Verification items for the finished model (mm, model axes). A direction names the side the tool comes from. Round coordinates to 2 decimals unless told otherwise and drop trailing zeros. Write each loop counter-clockwise with the first axis right and the second up, starting at its lowest first coordinate (ties: lowest second). Pieces come first, ordered by that corner, then holes. Notation, with made-up numbers: M -22.75,38.25 L -11.75,38.25 A18 cw -11.75,45.25 Z; hole C 9,23.5 d9. An arc over 180 degrees is marked long. Write each question's results on one line, items separated by ' | '.
from build123d import *

# Parameters (mm, degrees)
ESQUISSE1_W             = 55
ESQUISSE1_H             = 26
BOSS_EXTRU_1_DEPTH      = 25
ENL_V_MAT_EXTRU_1_REACH = 49.007
ESQUISSE2_W             = 10
ESQUISSE2_H             = 2
ENL_V_MAT_EXTRU_5_REACH = 64.857
ESQUISSE5_R             = 2.5
ESQUISSE5_W             = 26
ESQUISSE5_H             = 3.5


with BuildPart() as part:
    # Esquisse1 → Boss.-Extru.1 (new body)
    with BuildSketch(Plane(origin=(0, 0, 0), x_dir=(1, 0, 0), z_dir=(0, 1, 0))):
        with Locations((2.643338954, -4.351180438)):
            Rectangle(ESQUISSE1_W, ESQUISSE1_H)
    extrude(amount=BOSS_EXTRU_1_DEPTH)

    # Esquisse2 → Enlèv. mat.-Extru.1 (cut, up to next)
    with BuildSketch(Plane.XY.offset(17.351180438), mode=Mode.PRIVATE) as enl_v_mat_extru_1_sk1:
        with Locations((19.143338954, 16)):
            Rectangle(ESQUISSE2_W, ESQUISSE2_H)
    enl_v_mat_extru_1_tool1 = extrude(enl_v_mat_extru_1_sk1.sketch, amount=-ENL_V_MAT_EXTRU_1_REACH, mode=Mode.PRIVATE) & part.part
    # Esquisse2 → Enlèv. mat.-Extru.1 (cut, up to next)
    with BuildSketch(Plane.XY.offset(17.351180438), mode=Mode.PRIVATE) as enl_v_mat_extru_1_sk2:
        with Locations((-6.856661046, 16)):
            Rectangle(ESQUISSE2_W, ESQUISSE2_H)
    enl_v_mat_extru_1_tool2 = extrude(enl_v_mat_extru_1_sk2.sketch, amount=-ENL_V_MAT_EXTRU_1_REACH, mode=Mode.PRIVATE) & part.part
    add(enl_v_mat_extru_1_tool1.solids().sort_by_distance((19.143339, 16, 17.35118))[0], mode=Mode.SUBTRACT)
    add(enl_v_mat_extru_1_tool2.solids().sort_by_distance((-6.856661, 16, 17.35118))[0], mode=Mode.SUBTRACT)

    # Esquisse5 → Enlèv. mat.-Extru.5 (cut, up to next)
    with BuildSketch(Plane(origin=(30.143338954, 0, 0), x_dir=(0, 0, -1), z_dir=(1, 0, 0)), mode=Mode.PRIVATE) as enl_v_mat_extru_5_sk1:
        with Locations((-4.351180438, 9)):
            Circle(ESQUISSE5_R)
    enl_v_mat_extru_5_tool1 = extrude(enl_v_mat_extru_5_sk1.sketch, amount=-ENL_V_MAT_EXTRU_5_REACH, mode=Mode.PRIVATE) & part.part
    # Esquisse5 → Enlèv. mat.-Extru.5 (cut, up to next)
    with BuildSketch(Plane(origin=(30.143338954, 0, 0), x_dir=(0, 0, -1), z_dir=(1, 0, 0)), mode=Mode.PRIVATE) as enl_v_mat_extru_5_sk2:
        with BuildLine():
            Line((-17.351180438, 25), (8.648819562, 25))
            add(Edge.make_bspline(
                [(-17.351180438, 25), (-4.586883511, 15.502643884), (8.648819562, 25)],
                knots=[0, 0, 0, 1, 1, 1], degree=2))
        make_face()
    enl_v_mat_extru_5_tool2 = extrude(enl_v_mat_extru_5_sk2.sketch, amount=-ENL_V_MAT_EXTRU_5_REACH, mode=Mode.PRIVATE) & part.part
    # Esquisse5 → Enlèv. mat.-Extru.5 (cut, up to next)
    with BuildSketch(Plane(origin=(30.143338954, 0, 0), x_dir=(0, 0, -1), z_dir=(1, 0, 0)), mode=Mode.PRIVATE) as enl_v_mat_extru_5_sk3:
        with Locations((-4.351180438, 1.75)):
            Rectangle(ESQUISSE5_W, ESQUISSE5_H)
    enl_v_mat_extru_5_tool3 = extrude(enl_v_mat_extru_5_sk3.sketch, amount=-ENL_V_MAT_EXTRU_5_REACH, mode=Mode.PRIVATE) & part.part
    add(enl_v_mat_extru_5_tool1.solids().sort_by_distance((30.143339, 9, 4.35118))[0], mode=Mode.SUBTRACT)
    add(enl_v_mat_extru_5_tool2.solids().sort_by_distance((30.143339, 23.100529, 4.398321))[0], mode=Mode.SUBTRACT)
    add(enl_v_mat_extru_5_tool3.solids().sort_by_distance((30.143339, 1.75, 4.35118))[0], mode=Mode.SUBTRACT)


solid = part.part
1) Sectioned sample at C-C, the plane x = 16. Count the separate pieces of the cut face and the enclosed holes in it, and give its area (3 significant figures).
Calculated:
separate pieces: 2 | enclosed holes: 1 | area: 405 mm²
2) Sectioned sample at A-A, the plane y = 9. Record the cut outline in (x, z), and give its area (4 significant figures).
Calculated:
outline: M -24.86,-8.65 L 30.14,-8.65 L 30.14,1.85 L -24.86,1.85 Z; M -24.86,6.85 L 30.14,6.85 L 30.14,17.35 L -24.86,17.35 Z | area: 1,155 mm²
3) Draft check along X on faces 1 (the flat face through (-24.857, 12, 5)), 2 (the flat face through (-7, 17, 5)), 3 (the cylindrical face through (3.03, 6.56, 4.89)), 4 (the flat face through (30.143, 12, 5)). Enter one of: pulls with the +X half, pulls with the -X half, needs draft (parallel to the pull), parting line crosses it, or undercut.
Calculated:
face 1: pulls with the -X half | face 2: undercut | face 3: needs draft | face 4: pulls with the +X half
4) Access from +Z, -Z, +X, -X, +Y, -Y to the whole of each face (thin tool, end or side, straight path). Record for faces 5 (the flat face through (3, 3.5, 5)), 6 (the flat face through (-11.857, 16, 5)).
Calculated:
face 5: +Z, -Z, +X, -X, -Y | face 6: +Z, -Z
5) Depth check by flat-ended pin: P1, Ø11, axis at x = -4.5, z = 0, coming from the +Y side; P2, Ø10, axis at x = 24, z = 10.5, coming from the +Y side; P3, Ø5, axis at x = 21, z = 10.5, coming from the +Y side. Enter the tip coordinate at first touch or a pass-through.
Calculated:
P1: stops at y = 23.01 | P2: stops at y = 23.72 | P3: stops at y = 22.32
6) Sectioned sample at B-B, the plane y = 15.75. Record the cut outline in (x, z), and give its area (3 significant figures).
Calculated:
outline: M -24.86,-8.65 L -11.86,-8.65 L -11.86,17.35 L -24.86,17.35 Z; M -1.86,-8.65 L 14.14,-8.65 L 14.14,17.35 L -1.86,17.35 Z; M 24.14,-8.65 L 30.14,-8.65 L 30.14,17.35 L 24.14,17.35 Z | area: 910 mm²
7) Material ranges on line 1 (Y direction, x = -6.5, z = 2.75); line 2 (Y direction, x = 21, z = 4); line 3 (Z direction, x = -5.5, y = 9.5), recorded low to high. Write a range as [from, to].
Calculated:
line 1: y = [3.5, 7.08], [10.92, 15], [17, 20.33] | line 2: y = [3.5, 6.52], [11.48, 15], [17, 20.26] | line 3: z = [-8.65, 1.9], [6.8, 17.35]
